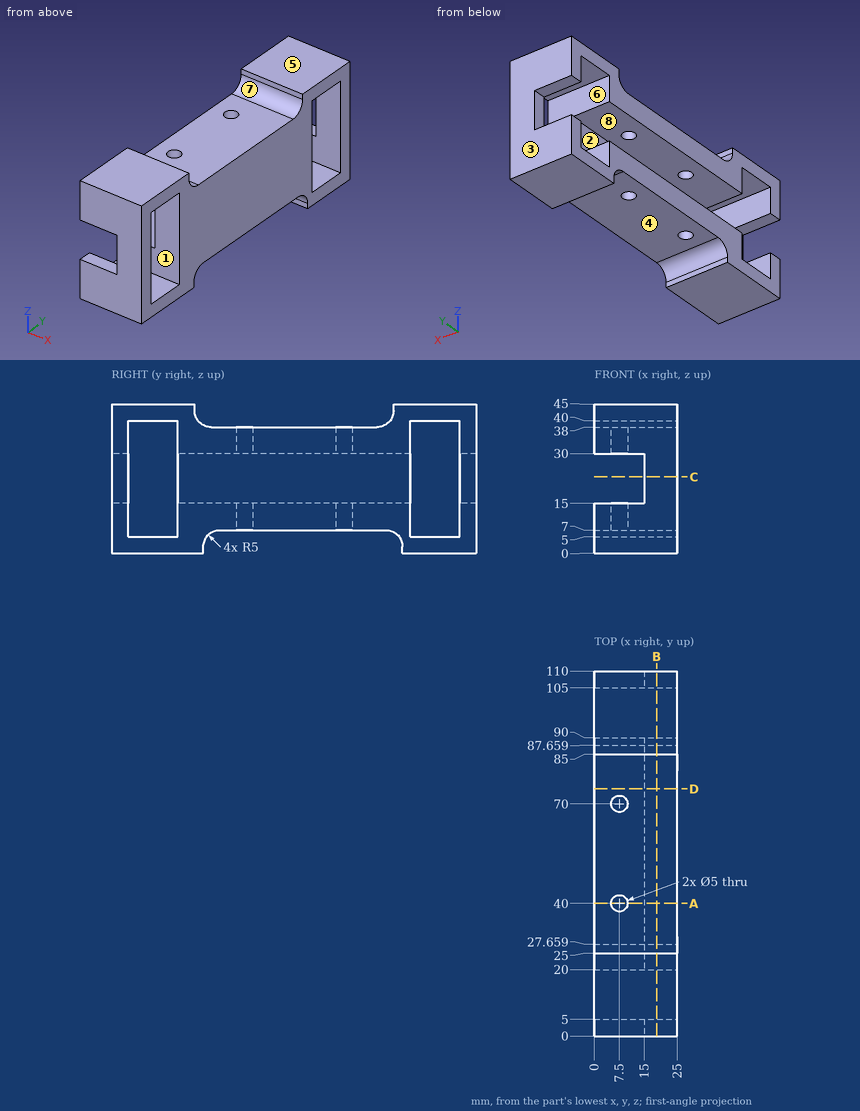
Could you check a few things on this drawing? It's one solid part, dimensions in mm from its lowest x, y, z. A direction names the side the tool comes from. Give positions to 0.01 mm unless a question says otherwise; leave off trailing zeros. Write each loop counter-clockwise with the first axis right and the second up, starting at its lowest first coordinate (ties: lowest second). Pieces come first, ordered by that corner, then holes. Notation, with made-up numbers: (7.25, 10.25) -> (63.25, 10.25) arc R24 cw to (63.25, 31.25) -> close; hole circle Ø9 at (70, 6.25). An arc over 180 degrees is marked (long way). Answer as CSV lines item,"result". Start each with the question number.
(1) I'm going to push flat-ended pins straight in: pin 1 Ø1.5 at (x, y) = (15, 30) entering from +Z; pin 2 Ø3 at (x, y) = (17.5, 75.5) entering from +Z; pin 3 Ø2 at (y, z) = (28, 22.5) entering from -X. Where does each tip first touch, or does it pass through?
(2) Which directions (+Z, -Z, +X, -X, +Y, -Y) give clear straight access to the entire face, cutting with the end or side of a thin tool? Please do the marked faces 4, 5, 6, 7 and 8.
(3) Please list where these lines run through material, in increasing order: line 1 (Y direction, x = 7.5, z = 32); line 2 (Y direction, x = 3.5, z = 35.5); line 3 (Z direction, x = 11.25, y = 103).
(4) If we section it at A-A, the plane y = 40: Write out the boundary of the cut face in (x, z).
(5) If we section it at D-D, the plane y = 74.5: Write out the boundary of the cut face in (x, z), and give its area (3 significant figures).
(6) If we section it at B-B, the plane x = 18.75: Write out the boundary of the cut face in (y, z).
(7) If we section it at C-C, the plane z = 23: Write out the boundary of the cut face in (x, y), and give its area (3 significant figures).
(8) If we mould it in two halves opening along Y, with no side actions, what happens to the marked faces 1, 2 and 3? For each: +Y half, -Y half, draft (parallel to the pull), parting line (faces both ways), or undercut.
Answer list:
1,pin 1,"z = 38.06"
1,pin 2,"z = 38"
1,pin 3,"x = 15"
2,face 4,"-Z, +X, -X"
2,face 5,"+Z, +X, -X, +Y, -Y"
2,face 6,"+X, -X"
2,face 7,"+Z, +X, -X"
2,face 8,"-X, +Y, -Y"
3,line 1,"0 to 5, 20 to 37.5, 42.5 to 67.5, 72.5 to 90, 105 to 110"
3,line 2,"0 to 5, 20 to 90, 105 to 110"
3,line 3,"0 to 5, 40 to 45"
4,outline,"(0, 7) -> (5, 7) -> (5, 15) -> (0, 15) -> close; (0, 30) -> (5, 30) -> (5, 38) -> (0, 38) -> close; (10, 7) -> (25, 7) -> (25, 38) -> (10, 38) -> (10, 30) -> (15, 30) -> (15, 15) -> (10, 15) -> close"
5,outline,"(0, 7) -> (25, 7) -> (25, 38) -> (0, 38) -> (0, 30) -> (15, 30) -> (15, 15) -> (0, 15) -> close"
5,area,"550 mm^2"
6,outline,"(0, 0) -> (27.66, 0) -> (27.66, 2) arc R5 cw to (32.66, 7) -> (82.66, 7) arc R5 cw to (87.66, 2) -> (87.66, 0) -> (110, 0) -> (110, 45) -> (85, 45) -> (85, 43) arc R5 cw to (80, 38) -> (30, 38) arc R5 cw to (25, 43) -> (25, 45) -> (0, 45) -> close; hole (5, 5) -> (20, 5) -> (20, 40) -> (5, 40) -> close; hole (90, 5) -> (105, 5) -> (105, 40) -> (90, 40) -> close"
7,outline,"(15, 0) -> (25, 0) -> (25, 5) -> (15, 5) -> close; (15, 20) -> (25, 20) -> (25, 90) -> (15, 90) -> close; (15, 105) -> (25, 105) -> (25, 110) -> (15, 110) -> close"
7,area,"800 mm^2"
8,face 1,"undercut"
8,face 2,"draft"
8,face 3,"+Y half"
